Could you check a few things on this model? Use its own coordinates, in mm. Face numbers are marked on the shaded views. A direction names the side the tool comes from. Give positions to 0.01 mm unless a question says otherwise; leave off trailing zeros. Write each loop counter-clockwise with the first axis right and the second up, starting at its lowest first coordinate (ties: lowest second). Pieces come first, ordered by that corner, then holes. Notation, with made-up numbers: (58, -30.5) -> (96, -30.5) arc R17 cw to (96, -3.5) -> close; hole circle Ø8 at (26, 87.5). An arc over 180 degrees is marked (long way). One line per question, with ' | ' between items.
from build123d import *

# Parameters (mm, degrees)
BOSS_EXTRUDE1_DEPTH     = 12
SKETCH2_R               = 8.9
SKETCH2_R_2             = 2
SKETCH2_R_3             = 0.8
BOSS_EXTRUDE2_DEPTH     = 3
SKETCH4_R               = 2.5
SKETCH4_R_2             = 2.8
CUT_EXTRUDE1_DEPTH      = 0.8
SKETCH9_R               = 2
CUT_EXTRUDE4_DEPTH      = 3
SKETCH10_R              = 2.5
CUT_EXTRUDE5_DEPTH      = 0.8
MIRROR3_COPY_1_SKETCH_R = 2.5
MIRROR3_COPY_1_DEPTH    = 0.8
CUT_EXTRUDE3_DEPTH      = 9
SKETCH5_W               = 6
SKETCH5_H               = 6
SKETCH5_R               = 2
SKETCH5_H_2             = 11.4
BOSS_EXTRUDE3_DEPTH     = 1.5
SKETCH6_R               = 2.5
SKETCH6_W               = 6
SKETCH6_H               = 11.4
CUT_EXTRUDE2_DEPTH      = 0.8
SKETCH11_R              = 2
CUT_EXTRUDE6_DEPTH      = 0.8
CUT_EXTRUDE7_DEPTH      = 2.25
SKETCH13_R              = 2
CUT_EXTRUDE8_DEPTH      = 3
SKETCH14_R              = 2.5
CUT_EXTRUDE9_DEPTH      = 0.8


with BuildPart() as part:
    # Sketch1 → Boss-Extrude1 (new body, symmetric)
    with BuildSketch(Plane.XY):
        Polygon((8, 18), (-8, 18), (-10.5, 14.15), (-10.5, -14.15), (-8, -18), (8, -18), (10.5, -14.15), (10.5, 14.15), align=None)
    extrude(amount=BOSS_EXTRUDE1_DEPTH, both=True)

    # Sketch2 → Boss-Extrude2 (add)
    with BuildSketch(Plane.XY.offset(12)):
        with Locations((0, -9.1)):
            Circle(SKETCH2_R)
        with Locations((0, -15.3)):
            Circle(SKETCH2_R_2, mode=Mode.SUBTRACT)
        with Locations((-4.384062043, -13.484062043)):
            Circle(SKETCH2_R_3, mode=Mode.SUBTRACT)
        with Locations((4.384062043, -13.484062043)):
            Circle(SKETCH2_R_3, mode=Mode.SUBTRACT)
        with Locations((6.2, -9.1)):
            Circle(SKETCH2_R_2, mode=Mode.SUBTRACT)
        with Locations((4.384062043, -4.715937957)):
            Circle(SKETCH2_R_3, mode=Mode.SUBTRACT)
        with Locations((0, -2.9)):
            Circle(SKETCH2_R_2, mode=Mode.SUBTRACT)
        with Locations((-4.384062043, -4.715937957)):
            Circle(SKETCH2_R_3, mode=Mode.SUBTRACT)
        with Locations((-6.2, -9.1)):
            Circle(SKETCH2_R_2, mode=Mode.SUBTRACT)
    extrude(amount=BOSS_EXTRUDE2_DEPTH)

    # Sketch4 → Cut-Extrude1 (cut)
    with BuildSketch(Plane.XY.offset(15)):
        with Locations((0, -15.3)):
            Circle(SKETCH4_R)
        with Locations((0, -2.9)):
            Circle(SKETCH4_R)
        with Locations((-6.2, -9.1)):
            Circle(SKETCH4_R)
        with Locations((6.2, -9.1)):
            Circle(SKETCH4_R)
        with Locations((0, -9.1)):
            Circle(SKETCH4_R_2)
    extrude(amount=-CUT_EXTRUDE1_DEPTH, mode=Mode.SUBTRACT)

    # Sketch9 → Cut-Extrude4 (cut)
    with BuildSketch(Plane.XY.offset(12)):
        with Locations((0, 15)):
            Circle(SKETCH9_R)
        with Locations((6, 15)):
            Circle(SKETCH9_R)
        with Locations((-6, 15)):
            Circle(SKETCH9_R)
    cut_extrude4 = extrude(amount=-CUT_EXTRUDE4_DEPTH, mode=Mode.SUBTRACT)

    # Sketch10 → Cut-Extrude5 (cut)
    with BuildSketch(Plane.XY.offset(12)):
        with Locations((0, 15)):
            Circle(SKETCH10_R)
        with Locations((6, 15)):
            Circle(SKETCH10_R)
        with Locations((-6, 15)):
            Circle(SKETCH10_R)
    cut_extrude5 = extrude(amount=-CUT_EXTRUDE5_DEPTH, mode=Mode.SUBTRACT)

    # Mirror2: Cut-Extrude5 across plane
    add(cut_extrude5.mirror(Plane.XY.offset(10.5)), mode=Mode.SUBTRACT)

    # Mirror3: Cut-Extrude4, Cut-Extrude5 across plane
    add(cut_extrude4.mirror(Plane.XY), mode=Mode.SUBTRACT)
    add(cut_extrude5.mirror(Plane.XY), mode=Mode.SUBTRACT)

    # Mirror3 copy 1 sketch → Mirror3 copy 1 (cut)
    with BuildSketch(Plane.XY.offset(-9)):
        with Locations((0, 15)):
            Circle(MIRROR3_COPY_1_SKETCH_R)
        with Locations((6, 15)):
            Circle(MIRROR3_COPY_1_SKETCH_R)
        with Locations((-6, 15)):
            Circle(MIRROR3_COPY_1_SKETCH_R)
    extrude(amount=-MIRROR3_COPY_1_DEPTH, mode=Mode.SUBTRACT)

    # Sketch8 → Cut-Extrude3 (cut, symmetric)
    with BuildSketch(Plane.XY):
        with BuildLine():
            Line((8, 18), (-8, 18))
            Line((-8, 18), (-10.5, 14.15))
            Line((-10.5, 14.15), (-10.5, 12.5))
            Line((-10.5, 12.5), (-6, 12.5))
            ThreePointArc((-6, 12.5), (-4.881966011, 12.763932023), (-4, 13.5))
            Line((-4, 13.5), (4, 13.5))
            ThreePointArc((4, 13.5), (4.881966011, 12.763932023), (6, 12.5))
            Line((6, 12.5), (10.5, 12.5))
            Line((10.5, 12.5), (10.5, 14.15))
            Line((10.5, 14.15), (8, 18))
        make_face()
    extrude(amount=CUT_EXTRUDE3_DEPTH, both=True, mode=Mode.SUBTRACT)

    # Sketch5 → Boss-Extrude3 (add)
    with BuildSketch(Plane(origin=(10.5, 0, 0), x_dir=(0, 0, -1), z_dir=(1, 0, 0))):
        with Locations((-6, -10)):
            Rectangle(SKETCH5_W, SKETCH5_H)
        with Locations((-6, -10)):
            Circle(SKETCH5_R, mode=Mode.SUBTRACT)
        with Locations((6, -0.5)):
            Rectangle(SKETCH5_W, SKETCH5_H_2)
        with Locations((-6, 9)):
            Rectangle(SKETCH5_W, SKETCH5_H)
        with Locations((-6, 9)):
            Circle(SKETCH5_R, mode=Mode.SUBTRACT)
        with Locations((6, 9)):
            Rectangle(SKETCH5_W, SKETCH5_H)
        with Locations((6, 9)):
            Circle(SKETCH5_R, mode=Mode.SUBTRACT)
        with Locations((6, -10)):
            Rectangle(SKETCH5_W, SKETCH5_H)
        with Locations((6, -10)):
            Circle(SKETCH5_R, mode=Mode.SUBTRACT)
    boss_extrude3 = extrude(amount=BOSS_EXTRUDE3_DEPTH)

    # Sketch6 → Cut-Extrude2 (cut)
    with BuildSketch(Plane(origin=(12, 0, 0), x_dir=(0, 0, -1), z_dir=(1, 0, 0))):
        with Locations((-6, -10)):
            Circle(SKETCH6_R)
        with Locations((-6, 9)):
            Circle(SKETCH6_R)
        with Locations((6, 9)):
            Circle(SKETCH6_R)
        with Locations((6, -10)):
            Circle(SKETCH6_R)
        with Locations((6, -0.5)):
            Rectangle(SKETCH6_W, SKETCH6_H)
    cut_extrude2 = extrude(amount=-CUT_EXTRUDE2_DEPTH, mode=Mode.SUBTRACT)

    # Sketch11 → Cut-Extrude6 (cut)
    with BuildSketch(Plane(origin=(10.5, 0, 0), x_dir=(0, 0, -1), z_dir=(1, 0, 0))):
        with Locations((0, 9)):
            Circle(SKETCH11_R)
        with Locations((0, -10)):
            Circle(SKETCH11_R)
    cut_extrude6 = extrude(amount=-CUT_EXTRUDE6_DEPTH, mode=Mode.SUBTRACT)

    # Mirror4: Boss-Extrude3, Cut-Extrude2, Cut-Extrude6 across plane
    add(boss_extrude3.mirror(Plane(origin=(0, 0, 0), x_dir=(0, 0, 1), z_dir=(1, 0, 0))))
    add(cut_extrude2.mirror(Plane(origin=(0, 0, 0), x_dir=(0, 0, 1), z_dir=(1, 0, 0))), mode=Mode.SUBTRACT)
    add(cut_extrude6.mirror(Plane(origin=(0, 0, 0), x_dir=(0, 0, 1), z_dir=(1, 0, 0))), mode=Mode.SUBTRACT)

    # Sketch12 → Cut-Extrude7 (cut)
    with BuildSketch(Plane(origin=(0, 0, 9), x_dir=(-1, 0, 0), z_dir=(0, 0, -1))):
        with BuildLine():
            Line((-6, 12.5), (-10.5, 12.5))
            Line((-10.5, 12.5), (-10.5, 12))
            Line((-10.5, 12), (-6, 12))
            ThreePointArc((-6, 12), (-4.5, 12.401923789), (-3.401923789, 13.5))
            Line((-3.401923789, 13.5), (-4, 13.5))
            ThreePointArc((-4, 13.5), (-4.881966011, 12.763932023), (-6, 12.5))
        make_face()
        with BuildLine():
            Line((3.401923789, 13.5), (4, 13.5))
            ThreePointArc((4, 13.5), (4.881966011, 12.763932023), (6, 12.5))
            Line((6, 12.5), (10.5, 12.5))
            Line((10.5, 12.5), (10.5, 12))
            Line((10.5, 12), (6, 12))
            ThreePointArc((6, 12), (4.5, 12.401923789), (3.401923789, 13.5))
        make_face()
    cut_extrude7 = extrude(amount=CUT_EXTRUDE7_DEPTH, mode=Mode.SUBTRACT)

    # Mirror5: Cut-Extrude7 across plane
    add(cut_extrude7.mirror(Plane.XY), mode=Mode.SUBTRACT)

    # Sketch13 → Cut-Extrude8 (cut)
    with BuildSketch(Plane(origin=(0, 0, -12), x_dir=(-1, 0, 0), z_dir=(0, 0, -1))):
        with Locations((0, -9.1)):
            Circle(SKETCH13_R)
        with Locations((6, -9.1)):
            Circle(SKETCH13_R)
        with Locations((-6, -9.1)):
            Circle(SKETCH13_R)
    extrude(amount=-CUT_EXTRUDE8_DEPTH, mode=Mode.SUBTRACT)

    # Sketch14 → Cut-Extrude9 (cut)
    with BuildSketch(Plane(origin=(0, 0, -12), x_dir=(-1, 0, 0), z_dir=(0, 0, -1))):
        with Locations((0, -9.1)):
            Circle(SKETCH14_R)
        with Locations((6, -9.1)):
            Circle(SKETCH14_R)
        with Locations((-6, -9.1)):
            Circle(SKETCH14_R)
    extrude(amount=-CUT_EXTRUDE9_DEPTH, mode=Mode.SUBTRACT)


solid = part.part
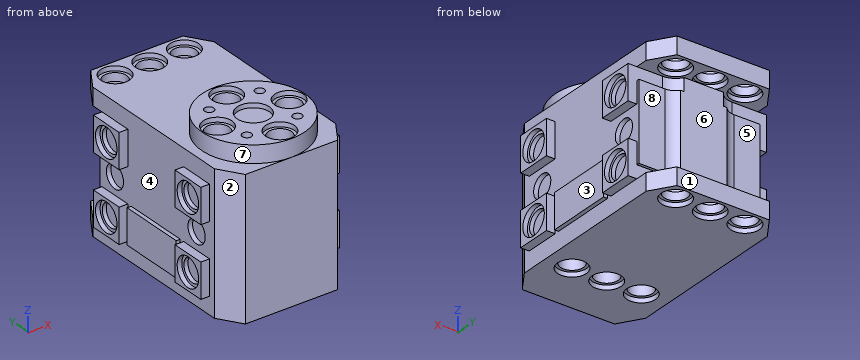
Q1. Imagine slicing it at D-D on y = -15.3. Please give me the cut outline in (x, z), and give its area (3 significant figures).
Answer below:
outline: (-9.75, -12) -> (9.75, -12) -> (9.75, 12) -> (6.39, 12) -> (6.39, 15) -> (2.5, 15) -> (2.5, 14.2) -> (2, 14.2) -> (2, 12) -> (-2, 12) -> (-2, 14.2) -> (-2.5, 14.2) -> (-2.5, 15) -> (-6.39, 15) -> (-6.39, 12) -> (-9.75, 12) -> close | area: 494 mm^2
Q2. On a 3-axis mill with a long thin cutter (end or side, diameter ignored), from which of +Z, -Z, +X, -X, +Y, -Y can I reach the whole of each face in a straight line? I mean the marked faces 5, 6, 7 and 8. Say none if no direction works.
Answer below:
face 5: -X, +Y | face 6: +X, -X, +Y | face 7: +Z | face 8: +X, +Y
Q3. If I drill on line 1 along Y through (x, z) = (0, -11.8); line 2 along Z through (x, y) = (10.65, -10); line 3 along Z through (x, y) = (9.25, 14), over which ranges is the centre line in solid material (lowest first)?
Answer below:
line 1: y = -18 to -11.6, -6.6 to 12.5, 17.5 to 18 | line 2: z = -9 to -8, -4 to -3, 3 to 4, 8 to 9 | line 3: z = -12 to -9, 9 to 12
Q4. Imagine slicing it at B-B on x = -0.75. Count the separate pieces of the cut face and the enclosed holes in it, and give its area (3 significant figures).
Answer below:
separate pieces: 3 | enclosed holes: 0 | area: 770 mm^2
Q5. If we mould it in two halves opening along Y, with no side actions, what happens to the marked faces 1, 2, 3 and 4? For each: +Y half, -Y half, draft (parallel to the pull), parting line (faces both ways), or undercut.
Answer below:
face 1: +Y half | face 2: -Y half | face 3: undercut | face 4: undercut
Q6. Imagine slicing it at A-A on y = 1. Please give me the cut outline in (x, z), and give its area (3 significant figures).
Answer below:
outline: (-11.2, -9) -> (-10.5, -9) -> (-10.5, -12) -> (10.5, -12) -> (10.5, -9) -> (11.2, -9) -> (11.2, -3) -> (10.5, -3) -> (10.5, 12) -> (-10.5, 12) -> (-10.5, -3) -> (-11.2, -3) -> close | area: 512 mm^2
Q7. Will these pins go through, and if not, where does the flat tip stop? pin 1 (2.5 mm diameter, centred on y = 9, z = 6, fed in from -X); pin 2 (3 mm diameter, centred on x = 1.5, y = 14, fed in from +Z); pin 3 (2.5 mm diameter, centred on x = -0.5, y = -16, fed in from +Z).
Answer below:
pin 1: stops at x = -10.5 | pin 2: stops at z = 12 | pin 3: stops at z = 14.2
